For this review, take the finished solid that the model builds, in its own axes (mm). Round coordinates to 2 decimals unless told otherwise and drop trailing zeros. Write each loop counter-clockwise with the first axis right and the second up, starting at its lowest first coordinate (ties: lowest second). Pieces come first, ordered by that corner, then holes. Notation, with made-up numbers: (-3, 84) -> (37, 84) arc R22 ccw to (37, 116) -> close; hole circle Ø10 at (40.25, 53). An arc over 180 degrees is marked (long way). Write each question's results on one line, items separated by ' | '. Start each with the question number.
Item 1: Add section C-C (x = 111). State the section outline as (y, z) points, plus the area to 3 significant figures.
Item 2: To check wall thickness, follow line 1 along Y through (x, z) = (0, 241.5); line 2 along Z through (x, y) = (12, 50); line 3 along Z through (x, y) = (-6.5, 30). State the ranges of each line that lie inside material, in increasing order.
Item 3: Add section B-B (y = 38.1). State the section outline as (x, z) points.
Item 4: Clearance check with a flat-ended pin moving along its axis: pin 1 (2 mm diameter, centred on x = -183.5, y = 56, fed in from +Z). State where the tip first meets the part, or that it passes through.
Item 5: Add section A-A (x = 0). State the section outline as (y, z) points, plus the area to 3 significant figures.
from build123d import *

# Parameters (mm, degrees)
BOSS_EXTRUDE1_DEPTH = 76.2
SKETCH12_R          = 7.5
CUT_EXTRUDE1_DEPTH  = 254


with BuildPart() as part:
    # Sketch1 → Boss-Extrude1 (new body)
    with BuildSketch(Plane(origin=(0, 0, 0), x_dir=(1, 0, 0), z_dir=(0, 1, 0))):
        with BuildLine():
            ThreePointArc((275.021699517, -216.577215773), (0, -238), (-275.021699517, -216.577215773))
            Line((-275.021699517, -216.577215773), (-275.021699517, -231.577215773))
            ThreePointArc((-275.021699517, -231.577215773), (0, -253), (275.021699517, -231.577215773))
            Line((275.021699517, -231.577215773), (275.021699517, -216.577215773))
        make_face()
    extrude(amount=BOSS_EXTRUDE1_DEPTH)

    # Sketch12 → Cut-Extrude1 (cut, through all)
    with BuildSketch(Plane.XY):
        with Locations((0, 38.1)):
            Circle(SKETCH12_R)
    extrude(amount=CUT_EXTRUDE1_DEPTH, mode=Mode.SUBTRACT)


solid = part.part
Responses:
1) outline: (0, 234.53) -> (76.2, 234.53) -> (76.2, 249.53) -> (0, 249.53) -> close | area: 1,140 mm^2
2) line 1: y = 0 to 30.6, 45.6 to 76.2 | line 2: z = 237.96 to 252.96 | line 3: z = 237.99 to 252.99
3) outline: (-275.02, 216.58) arc R1776.05 cw to (-7.5, 237.98) -> (-7.5, 252.98) arc R1776.05 ccw to (-275.02, 231.58) -> close; (7.5, 237.98) arc R1776.05 cw to (275.02, 216.58) -> (275.02, 231.58) arc R1776.05 ccw to (7.5, 252.98) -> close
4) pin 1: stops at z = 243.6
5) outline: (0, 238) -> (30.6, 238) -> (30.6, 253) -> (0, 253) -> close; (45.6, 238) -> (76.2, 238) -> (76.2, 253) -> (45.6, 253) -> close | area: 918 mm^2
